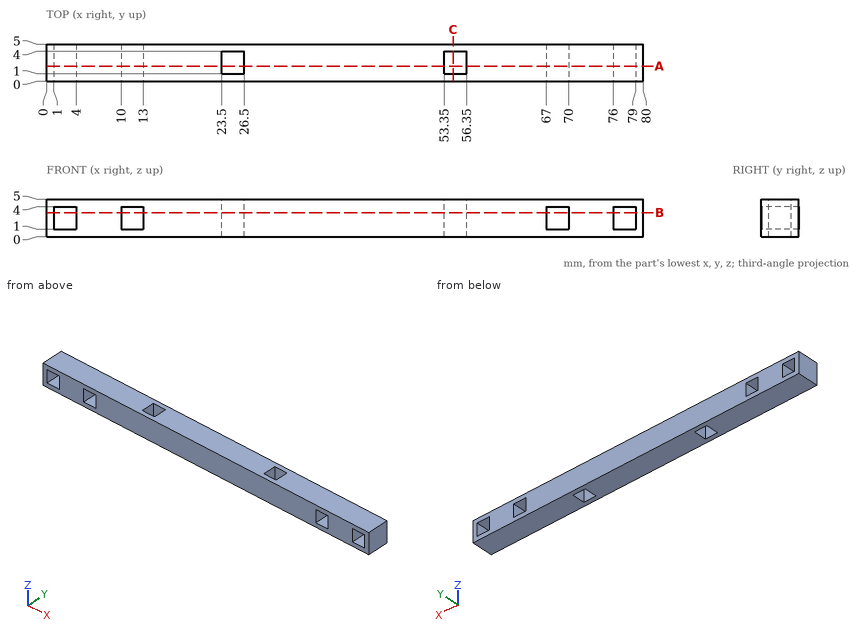
Source: three-view drawing plus pictorial views. Frame: mm from the lowest corner of the part. Give positions to 0.01 mm unless a question says otherwise; leave off trailing zeros. Write each loop counter-clockwise with the first axis right and the second up, starting at its lowest first coordinate (ties: lowest second). Pieces come first, ordered by that corner, then holes. Notation, with made-up numbers: (8.5, 87.25) - (56.5, 87.25) arc R24 cw to (56.5, 104.25) - close; hole circle Ø6 at (16.5, -17). An arc over 180 degrees is marked (long way). Write item = value, one per line. Start each with the question number.
1. First-contact query: pin 1 Ø1 at (y, z) = (0.5, 1) entering from -X. Flat tip, straight axial feed; report the tip coordinate or a pass-through.
2. Section query A-A, the plane y = 2.05. Output: boundary loops of the cut face in (x, z), then the cut area to 3 significant figures.
3. Section query C-C, the plane x = 54.5. Output: boundary loops of the cut face in (y, z), then the cut area to 3 significant figures.
4. Ray query, L1, parallel to X at y = 4.55, z = 2.75; L2, parallel to X at y = 1.9, z = 0.5; L3, parallel to Z at x = 3.5, y = 2. Return the intervals inside material, ascending.
5. Section query B-B, the plane z = 3.2. Output: boundary loops of the cut face in (x, y).
Check sheet entries:
q1.pin_1 = 0
q2.outline = (0, 0) - (23.5, 0) - (23.5, 5) - (0, 5) - close; (26.5, 0) - (53.35, 0) - (53.35, 5) - (26.5, 5) - close; (56.35, 0) - (80, 0) - (80, 5) - (56.35, 5) - close; hole (1, 1) - (4, 1) - (4, 4) - (1, 4) - close; hole (10, 1) - (13, 1) - (13, 4) - (10, 4) - close; hole (67, 1) - (70, 1) - (70, 4) - (67, 4) - close; hole (76, 1) - (79, 1) - (79, 4) - (76, 4) - close
q2.area = 334 mm2
q3.outline = (0, 0) - (1, 0) - (1, 5) - (0, 5) - close; (4, 0) - (5, 0) - (5, 5) - (4, 5) - close
q3.area = 10.0 mm2
q4.L1 = 0 to 1, 4 to 10, 13 to 67, 70 to 76, 79 to 80
q4.L2 = 0 to 23.5, 26.5 to 53.35, 56.35 to 80
q4.L3 = 0 to 1, 4 to 5
q5.outline = (0, 0) - (1, 0) - (1, 5) - (0, 5) - close; (4, 0) - (10, 0) - (10, 5) - (4, 5) - close; (13, 0) - (67, 0) - (67, 5) - (13, 5) - close; (70, 0) - (76, 0) - (76, 5) - (70, 5) - close; (79, 0) - (80, 0) - (80, 5) - (79, 5) - close; hole (23.5, 1) - (26.5, 1) - (26.5, 4) - (23.5, 4) - close; hole (53.35, 1) - (56.35, 1) - (56.35, 4) - (53.35, 4) - close
